```python
from build123d import *

# Parameters (mm, degrees)
SKETCH1_W           = 228.6762
SKETCH1_H           = 3.175
BOSS_EXTRUDE1_DEPTH = 355.6
SKETCH2_W           = 31.75
SKETCH2_H           = 10.16
CUT_EXTRUDE1_DEPTH  = 423.793383429
SKETCH3_W           = 345.44
SKETCH3_H           = 198.4375
CUT_EXTRUDE2_DEPTH  = 2.032
SKETCH4_W           = 345.44
SKETCH4_H           = 198.4375
BOSS_EXTRUDE2_DEPTH = 2.0066
BOSS_EXTRUDE3_DEPTH = 2.54
FILLET1_R           = 3.81
SKETCH7_R           = 17.4625
SKETCH7_R_2         = 15.875
CUT_EXTRUDE3_DEPTH  = 0.254
CUT_EXTRUDE4_DEPTH  = 0.254
SKETCH9_R           = 1.905
CUT_EXTRUDE5_DEPTH  = 0.254
BOSS_EXTRUDE4_START = 0.2286
SKETCH10_R          = 1.905
BOSS_EXTRUDE4_DEPTH = 0.2286
BOSS_EXTRUDE5_START = 0.2286
BOSS_EXTRUDE5_DEPTH = 0.2286
SKETCH13_R          = 1.905
BOSS_EXTRUDE6_DEPTH = 146.05
FILLET2_R           = 3.81


with BuildPart() as part:
    # Sketch1 → Boss-Extrude1 (new body)
    with BuildSketch(Plane(origin=(0, 0, 0), x_dir=(0, 0, -1), z_dir=(1, 0, 0))):
        with Locations((114.3381, 1.5875)):
            Rectangle(SKETCH1_W, SKETCH1_H)
    extrude(amount=BOSS_EXTRUDE1_DEPTH)

    # Sketch2 → Cut-Extrude1 (cut, through all)
    with BuildSketch(Plane(origin=(0, 0, 0), x_dir=(-1, 0, 0), z_dir=(0, -1, 0))):
        with Locations((-15.875, 223.5962)):
            Rectangle(SKETCH2_W, SKETCH2_H)
        with Locations((-339.725, 223.5962)):
            Rectangle(SKETCH2_W, SKETCH2_H)
    extrude(amount=-CUT_EXTRUDE1_DEPTH, mode=Mode.SUBTRACT)

    # Sketch3 → Cut-Extrude2 (cut)
    with BuildSketch(Plane.XZ):
        with Locations((177.8, -104.29875)):
            Rectangle(SKETCH3_W, SKETCH3_H)
    extrude(amount=-CUT_EXTRUDE2_DEPTH, mode=Mode.SUBTRACT)

    # Sketch4 → Boss-Extrude2 (add)
    with BuildSketch(Plane.XZ.offset(-2.032)):
        with Locations((177.8, -104.29875)):
            Rectangle(SKETCH4_W, SKETCH4_H)
    extrude(amount=BOSS_EXTRUDE2_DEPTH)

    # Sketch6 → Boss-Extrude3 (add)
    with BuildSketch(Plane(origin=(0, 3.175, 0), x_dir=(1, 0, 0), z_dir=(0, 1, 0))):
        Polygon((-0.254, 218.5162), (-0.254, 228.9302), (355.854, 228.9302), (355.854, 218.5162), (355.854, -0.254), (-0.254, -0.254), align=None)
    extrude(amount=BOSS_EXTRUDE3_DEPTH)

    # Fillet1
    fillet1_edges = [part.edges().sort_by_distance(p)[0] for p in [
        (355.6, 1.5875, 0),
        (0, 1.5875, 0),
        (355.854, 4.445, -228.9302),
        (-0.254, 4.445, -228.9302),
        (-0.254, 4.445, 0.254),
        (355.854, 4.445, 0.254),
    ]]
    fillet(fillet1_edges, radius=FILLET1_R)

    # Sketch7 → Cut-Extrude3 (cut)
    with BuildSketch(Plane(origin=(0, 5.715, 0), x_dir=(1, 0, 0), z_dir=(0, 1, 0))):
        with Locations(Location((177.8, 114.3381, 0), (0, 0, 270))):
            Circle(SKETCH7_R)
        with Locations(Location((177.8, 114.3381, 0), (0, 0, 270))):
            Circle(SKETCH7_R_2, mode=Mode.SUBTRACT)
    extrude(amount=-CUT_EXTRUDE3_DEPTH, mode=Mode.SUBTRACT)

    # Sketch8 → Cut-Extrude4 (cut)
    # profile 1 of 2: a face of its own
    with BuildSketch(Plane(origin=(0, 5.715, 0), x_dir=(1, 0, 0), z_dir=(0, 1, 0))):
        with BuildLine():
            Line((189.471398708, 110.4011), (186.550398708, 110.4011))
            ThreePointArc((186.550398708, 110.4011), (184.504960684, 110.974151087), (183.054971216, 112.52648314))
            Line((183.054971216, 112.52648314), (179.786995785, 109.664107496))
            Line((179.786995785, 109.664107496), (178.860958774, 110.721364327))
            Line((178.860958774, 110.721364327), (181.805633989, 113.300565668))
            Line((181.805633989, 113.300565668), (181.102738426, 114.103061816))
            Line((181.102738426, 114.103061816), (178.158063211, 111.523860475))
            Line((178.158063211, 111.523860475), (177.2320262, 112.581117305))
            Line((177.2320262, 112.581117305), (180.176701415, 115.160318646))
            Line((180.176701415, 115.160318646), (179.473805853, 115.962814795))
            Line((179.473805853, 115.962814795), (176.529130638, 113.383613454))
            Line((176.529130638, 113.383613454), (175.943285209, 114.052473416))
            Line((175.943285209, 114.052473416), (175.943285209, 110.4011))
            Line((175.943285209, 110.4011), (173.911285209, 110.4011))
            Line((173.911285209, 110.4011), (173.911285209, 116.2431))
            Line((173.911285209, 116.2431), (171.625285209, 116.2431))
            Line((171.625285209, 116.2431), (171.625285209, 118.2751))
            Line((171.625285209, 118.2751), (175.943285209, 118.2751))
            Line((175.943285209, 118.2751), (175.943285209, 114.738839507))
            Line((175.943285209, 114.738839507), (180.379856415, 118.624772442))
            Line((180.379856415, 118.624772442), (182.882189217, 115.767858068))
            ThreePointArc((182.882189217, 115.767858068), (184.328798892, 117.588402025), (186.550398708, 118.2751))
            Line((186.550398708, 118.2751), (189.471398708, 118.2751))
            Line((189.471398708, 118.2751), (189.471398708, 110.4011))
        make_face()
        with BuildLine():
            Line((187.439398708, 112.4331), (187.439398708, 116.2431))
            Line((187.439398708, 116.2431), (186.550398708, 116.2431))
            ThreePointArc((186.550398708, 116.2431), (184.645398708, 114.3381), (186.550398708, 112.4331))
            Line((186.550398708, 112.4331), (187.439398708, 112.4331))
        make_face(mode=Mode.SUBTRACT)
    # profile 2 of 2: a face of its own
    with BuildSketch(Plane(origin=(0, 5.715, 0), x_dir=(1, 0, 0), z_dir=(0, 1, 0))):
        Polygon((168.831285209, 116.2431), (168.831285209, 110.4011), (170.863285209, 110.4011), (170.863285209, 118.2751), (166.545285209, 118.2751), (166.545285209, 116.2431), align=None)
    extrude(amount=-CUT_EXTRUDE4_DEPTH, mode=Mode.SUBTRACT)

    # Sketch9 → Cut-Extrude5 (cut)
    # profile 1 of 3: a face of its own
    with BuildSketch(Plane.XZ):
        with Locations(Location((96.52, -212.4075, 0), (0, 0, 270))):
            Circle(SKETCH9_R)
    # profile 2 of 3: a face of its own
    with BuildSketch(Plane.XZ):
        with BuildLine():
            Line((163.597466716, -204.7875), (163.597466716, -214.4395))
            Line((163.597466716, -214.4395), (167.153466716, -214.4395))
            ThreePointArc((167.153466716, -214.4395), (169.995954467, -213.513569152), (171.747705751, -211.091080351))
            Line((171.747705751, -211.091080351), (177.435092391, -215.322094253))
            Line((177.435092391, -215.322094253), (181.43588491, -209.94417434))
            Line((181.43588491, -209.94417434), (181.43588491, -214.4395))
            Line((181.43588491, -214.4395), (187.023578862, -214.4395))
            Line((187.023578862, -214.4395), (187.023578862, -211.885215882))
            Line((187.023578862, -211.885215882), (184.074788764, -211.885215882))
            Line((184.074788764, -211.885215882), (184.074788764, -204.7875))
            Line((184.074788764, -204.7875), (181.43588491, -204.7875))
            Line((181.43588491, -204.7875), (181.43588491, -209.234781788))
            Line((181.43588491, -209.234781788), (180.463746146, -208.51157922))
            Line((180.463746146, -208.51157922), (177.292916042, -212.773852326))
            Line((177.292916042, -212.773852326), (176.395981379, -212.106596296))
            Line((176.395981379, -212.106596296), (179.566811483, -207.84432319))
            Line((179.566811483, -207.84432319), (178.117732485, -206.766310779))
            Line((178.117732485, -206.766310779), (174.946902382, -211.028583886))
            Line((174.946902382, -211.028583886), (174.049967719, -210.361327856))
            Line((174.049967719, -210.361327856), (177.220797822, -206.099054749))
            Line((177.220797822, -206.099054749), (175.771718825, -205.021042339))
            Line((175.771718825, -205.021042339), (171.948374325, -210.160434204))
            ThreePointArc((171.948374325, -210.160434204), (170.754145851, -206.400186171), (167.153466716, -204.7875))
            Line((167.153466716, -204.7875), (163.597466716, -204.7875))
        make_face()
        with BuildLine():
            Line((166.391466716, -211.6455), (167.153466716, -211.6455))
            ThreePointArc((167.153466716, -211.6455), (169.185466716, -209.6135), (167.153466716, -207.5815))
            Line((167.153466716, -207.5815), (166.391466716, -207.5815))
            Line((166.391466716, -207.5815), (166.391466716, -211.6455))
        make_face(mode=Mode.SUBTRACT)
    # profile 3 of 3: a face of its own
    with BuildSketch(Plane.XZ):
        Polygon((190.678788764, -204.7875), (188.03988491, -204.7875), (188.03988491, -209.234781788), (188.03988491, -209.94417434), (188.03988491, -214.4395), (193.627578862, -214.4395), (193.627578862, -211.885215882), (190.678788764, -211.885215882), align=None)
    extrude(amount=-CUT_EXTRUDE5_DEPTH, mode=Mode.SUBTRACT)

    # Sketch10 → Boss-Extrude4 (add)
    with BuildSketch(Plane.XZ.offset(-0.254).offset(BOSS_EXTRUDE4_START)):
        with Locations(Location((96.52, -212.4075, 0), (0, 0, 270))):
            Circle(SKETCH10_R)
    extrude(amount=-BOSS_EXTRUDE4_DEPTH)

    # Sketch12 → Boss-Extrude5 (add)
    with BuildSketch(Plane.XZ.offset(-0.254).offset(BOSS_EXTRUDE5_START)):
        Polygon((188.03988491, -204.7875), (188.03988491, -214.4395), (193.627578862, -214.4395), (193.627578862, -211.885215882), (190.678788764, -211.885215882), (190.678788764, -204.7875), align=None)
        with BuildLine():
            Line((167.153466716, -204.7875), (163.597466716, -204.7875))
            Line((163.597466716, -204.7875), (163.597466716, -214.4395))
            Line((163.597466716, -214.4395), (167.153466716, -214.4395))
            ThreePointArc((167.153466716, -214.4395), (169.995954467, -213.513569152), (171.747705751, -211.091080351))
            Line((171.747705751, -211.091080351), (177.435092391, -215.322094253))
            Line((177.435092391, -215.322094253), (181.43588491, -209.94417434))
            Line((181.43588491, -209.94417434), (181.43588491, -214.4395))
            Line((181.43588491, -214.4395), (187.023578862, -214.4395))
            Line((187.023578862, -214.4395), (187.023578862, -211.885215882))
            Line((187.023578862, -211.885215882), (184.074788764, -211.885215882))
            Line((184.074788764, -211.885215882), (184.074788764, -204.7875))
            Line((184.074788764, -204.7875), (181.43588491, -204.7875))
            Line((181.43588491, -204.7875), (181.43588491, -209.234781788))
            Line((181.43588491, -209.234781788), (180.463746146, -208.51157922))
            Line((180.463746146, -208.51157922), (177.292916042, -212.773852326))
            Line((177.292916042, -212.773852326), (176.395981379, -212.106596296))
            Line((176.395981379, -212.106596296), (179.566811483, -207.84432319))
            Line((179.566811483, -207.84432319), (178.117732485, -206.766310779))
            Line((178.117732485, -206.766310779), (174.946902382, -211.028583886))
            Line((174.946902382, -211.028583886), (174.049967719, -210.361327856))
            Line((174.049967719, -210.361327856), (177.220797822, -206.099054749))
            Line((177.220797822, -206.099054749), (175.771718825, -205.021042339))
            Line((175.771718825, -205.021042339), (171.948374325, -210.160434204))
            ThreePointArc((171.948374325, -210.160434204), (170.754145851, -206.400186171), (167.153466716, -204.7875))
        make_face()
    extrude(amount=-BOSS_EXTRUDE5_DEPTH)

    # Sketch13 → Boss-Extrude6 (add, symmetric)
    with BuildSketch(Plane.ZY.offset(-177.8)):
        with BuildLine():
            Line((-227.129067699, -5.461), (-227.129067699, 0))
            Line((-227.129067699, 0), (-220.144067699, 0))
            Line((-220.144067699, 0), (-220.144067699, -5.461))
            ThreePointArc((-220.144067699, -5.461), (-223.636567699, -8.9535), (-227.129067699, -5.461))
        make_face()
        with Locations((-223.5962, -5.08)):
            Circle(SKETCH13_R, mode=Mode.SUBTRACT)
    extrude(amount=BOSS_EXTRUDE6_DEPTH, both=True)

    # Fillet2
    # the kernel refuses this fillet: 3.81 mm, written as the material it takes off along each edge
    with BuildSketch(Plane(origin=(364.991776656, 0, -218.5162), x_dir=(0, 1, 0), z_dir=(-1, 0, 0))) as fillet2_piece_1:
        with BuildLine():
            CenterArc((3.81, -3.756710662), FILLET2_R, 99.594068227, 80.405931773)
            Line((0, -3.756710662), (-0.0762, -3.756710662))
            Line((-0.0762, -3.756710662), (-0.0762, 0))
            Line((-0.0762, 0), (0, 0.0762))
            ThreePointArc((0, 0.0762), (1.5875, 0.0762), (3.1623, 0.075134213))
            Line((3.1623, 0.075134213), (3.175, 0))
        make_face()
    extrude(amount=41.141776656, mode=Mode.SUBTRACT)
    with BuildSketch(Plane(origin=(-9.391776656, 0, -218.5162), x_dir=(0, 1, 0), z_dir=(1, 0, 0))) as fillet2_piece_2:
        with BuildLine():
            CenterArc((3.81, 3.756710662), FILLET2_R, 180, 80.405931773)
            Line((0, 3.756710662), (-0.0762, 3.756710662))
            Line((-0.0762, 3.756710662), (-0.0762, 0))
            Line((-0.0762, 0), (0, -0.0762))
            ThreePointArc((0, -0.0762), (1.5875, -0.0762), (3.1623, -0.075134213))
            Line((3.1623, -0.075134213), (3.175, 0))
        make_face()
    extrude(amount=41.141776656, mode=Mode.SUBTRACT)


solid = part.part
```
Design review of the part built by this model. Coordinates are the model's own, in mm. A direction names the side the tool comes from. Give positions to 0.01 mm unless a question says otherwise; leave off trailing zeros. Order: outer loops, then holes, each group sorted by start corner. A loop starts at its lowest first (then second) coordinate and runs counter-clockwise, first axis right, second up. Notation, with made-up numbers: (4, 23) -> (62, 23) arc R10 cw to (62, 29) -> close; hole circle Ø9 at (-38, -17). An arc over 180 degrees is marked (long way). Write item = value, one per line. Start each with the question number.
(1) We need section A-A on z = -69.5. Write out the cut boundary in (x, y) (3 decimals), plus the area to 3 significant figures.
(2) We need section C-C on z = -123.5. Write out the cut boundary in (x, y) (3 decimals).
(3) For faces 1 (the face through (175.755, -8.953, -223.56)), 2 (the face through (323.85, -2, -223)), 3 (the face through (177, 0, -207)), 4 (the face through (31.75, -1, -223)), 5 (the face through (180, 5.715, -141)), list the 3-axis set-ups (+Z, -Z, +X, -X, +Y, -Y) from which the entire face can be reached by the end or side of a thin tool; tool diameter is ignored.
(4) To check wall thickness, follow line 1 along Z through (x, y) = (281, -5); line 2 along Z through (x, y) = (187.5, 0.75); line 3 along Y through (x, z) = (160, -110) (3 decimals). State the ranges of each line that lie inside material, in increasing order.
(5) For pin 1 (1.6 mm diameter, centred on x = 160, y = 1, fed in from -Z); pin 2 (2 mm diameter, centred on y = -0.5, z = -32.5, fed in from -X); pin 3 (11.5 mm diameter, centred on x = 173, z = -210.5, fed in from -Y), all flat-tipped, find the tip position at first contact; note any pin that passes through.
Numbers:
q1.outline = (-0.254, 3.175) -> (0, 3.175) -> (0, 0) -> (5.08, 0) -> (5.08, 0.025) -> (350.52, 0.025) -> (350.52, 0) -> (355.6, 0) -> (355.6, 3.175) -> (355.854, 3.175) -> (355.854, 5.715) -> (-0.254, 5.715) -> close
q1.area = 2,020 mm^2
q2.outline = (-0.254, 3.175) -> (0, 3.175) -> (0, 0) -> (5.08, 0) -> (5.08, 0.025) -> (350.52, 0.025) -> (350.52, 0) -> (355.6, 0) -> (355.6, 3.175) -> (355.854, 3.175) -> (355.854, 5.715) -> (192.666, 5.715) -> (192.666, 5.461) -> (190.764, 5.461) -> (190.764, 5.715) -> (164.836, 5.715) -> (164.836, 5.461) -> (162.934, 5.461) -> (162.934, 5.715) -> (-0.254, 5.715) -> close
q3.face_1 = +X, -X, -Y
q3.face_2 = -Z, +X, -Y
q3.face_3 = +Z, +X, -X, -Y
q3.face_4 = -Z, -X, -Y
q3.face_5 = +Z, -Z, +X, -X, +Y
q4.line_1 = -227.13 to -225.5, -221.69 to -220.14
q4.line_2 = -228.68 to 0
q4.line_3 = 0.025 to 5.715
q5.pin_1 = -228.68
q5.pin_2 = 0
q5.pin_3 = 0
